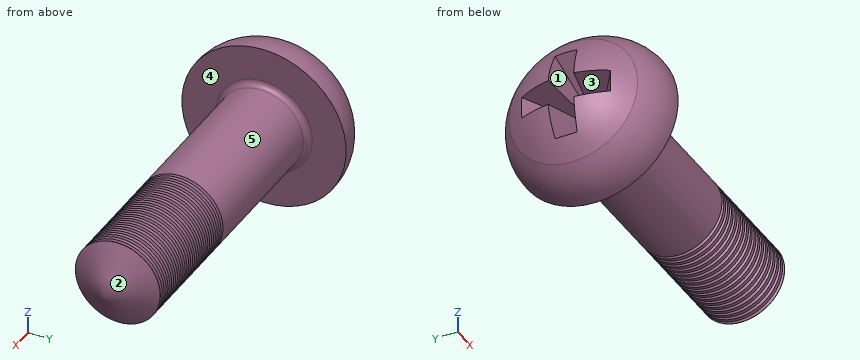
```python
from build123d import *

# Parameters (mm, degrees)
FILLET2_R        = 0.2
LPATTERN10_COUNT = 20
LPATTERN10_PITCH = 0.25


with BuildPart() as part:
    # Sketch1 → Revolve1 (revolve)
    with BuildSketch(Plane(origin=(0, 0, 0), x_dir=(1, 0, 0), z_dir=(0, 1, 0))):
        with BuildLine():
            Line((2.37, 1.5), (12.87, 1.5))
            Line((12.87, 1.5), (12.87, 0))
            Line((12.87, 0), (0, 0))
            ThreePointArc((0, 0), (0.224879408, 1.215980768), (0.869770135, 2.271109163))
            ThreePointArc((0.869770135, 2.271109163), (1.549177667, 2.754228297), (2.37, 2.9))
            Line((2.37, 2.9), (2.37, 1.5))
        make_face()
    revolve(axis=Axis((-13.629268293, 0, 0), (1, 0, 0)))

    # Fillet2
    fillet2_edges = [part.edges().sort_by_distance(p)[0] for p in [
        (2.37, 0, 1.5),
    ]]
    fillet(fillet2_edges, radius=FILLET2_R)

    # Sketch4 → Cut-Revolve1 (revolve, cut)
    with BuildSketch(Plane(origin=(0, 0, 0), x_dir=(1, 0, 0), z_dir=(0, 1, 0))):
        Polygon((13.603454633, 0), (13.603454633, 21), (0.745644347, 21), (12.87, 0), align=None)
    revolve(axis=Axis((4.782773752, 0, 0), (1, 0, 0)), mode=Mode.SUBTRACT)

    # Sketch2 → Cut-Loft1 section 0
    with BuildSketch(Plane(origin=(0, 0, 0), x_dir=(0, 0, -1), z_dir=(1, 0, 0)), mode=Mode.PRIVATE) as cut_loft1_s0:
        Polygon((-0.4625, 0.4625), (-1.85, 0.4625), (-1.85, -0.4625), (-0.4625, -0.4625), (-0.4625, -1.85), (0.4625, -1.85), (0.4625, -0.4625), (1.85, -0.4625), (1.85, 0.4625), (0.4625, 0.4625), (0.4625, 1.85), (-0.4625, 1.85), align=None)
    loft([Vertex(2.62, 0, 0), cut_loft1_s0.sketch], mode=Mode.SUBTRACT)

    # Sketch6 → Cut-Revolve10 (revolve, cut)
    with BuildSketch(Plane.XY):
        Polygon((7.87, 1.7), (7.995, 1.7), (7.995, 1.5), (7.9325, 1.391746825), (7.87, 1.5), align=None)
    cut_revolve10 = revolve(axis=Axis((10.774329131, 0, 0), (-1, 0, 0)), mode=Mode.SUBTRACT)

    # LPattern10: Cut-Revolve10 ×20
    with Locations(*[(i * LPATTERN10_PITCH, 0, 0) for i in range(1, LPATTERN10_COUNT)]):
        add(cut_revolve10, mode=Mode.SUBTRACT)


solid = part.part
```
The listing builds one solid part. Answer for the finished solid, in the listing's coordinates (mm). Face numbers are marked on the shaded views. A direction names the side the tool comes from. Round coordinates to 2 decimals unless told otherwise and drop trailing zeros. Loops run counter-clockwise (first coordinate to the right, second up) from the corner with the lowest first, then second, coordinate; pieces in that order, holes last.
Q1. Section A-A, the plane x = 5.25 is taken. Determine the outline of the cut face in (y, z), then the cut area to 3 significant figures.
Q2. Find the intervals of material crossed by line 1 (X direction, y = 0.55, z = 2.2); line 2 (Y direction, x = 7.5, z = 0.1); line 3 (Y direction, x = 7.5, z = -1.15), in increasing order.
Q3. Which of the six approach directions +Z, -Z, +X, -X, +Y, -Y give full straight-line access (tool end or side, diameter ignored) to the marked faces 1 and 2?
Q4. Given pin 1 Ø2 at (y, z) = (0, -2) entering from +X; pin 2 Ø1.5 at (x, z) = (5, 0.5) entering from -Y; pin 3 Ø1 at (y, z) = (0.5, -1.5) entering from -X, each flat-ended and moving along its own axis, determine where each tip first touches the part or whether it passes through.
Q5. For a pull along Z with two mould halves and no side action, classify the marked faces 3, 4 and 5 as released by +Z, released by -Z, zero draft, split by the parting line, or undercut.
Completed:
1. outline: circle Ø3 at (0, 0)
1. area: 7.07 mm2
2. line 1: x = 0.87 to 2.37
2. line 2: y = -1.5 to 1.5
2. line 3: y = -0.96 to 0.96
3. face 1: -X
3. face 2: +X
4. pin 1: stops at x = 12.29
4. pin 2: stops at y = -1.5
4. pin 3: stops at x = 0.18
5. face 3: undercut
5. face 4: zero draft
5. face 5: split by the parting line
